Can you work these out from the model? Positions are in its coordinate system, mm. Face numbers are marked on the shaded views. A direction names the side the tool comes from. Coordinates: 2 decimals unless noted, no trailing zeros. Order: outer loops, then holes, each group sorted by start corner. A loop starts at its lowest first (then second) coordinate and runs counter-clockwise, first axis right, second up. Notation, with made-up numbers: M 67,-24 L 86,-24 A32 cw 86,6 Z; hole C 0,-2 d4. An arc over 180 degrees is marked long. Answer as a JSON object with one key per item and string values.
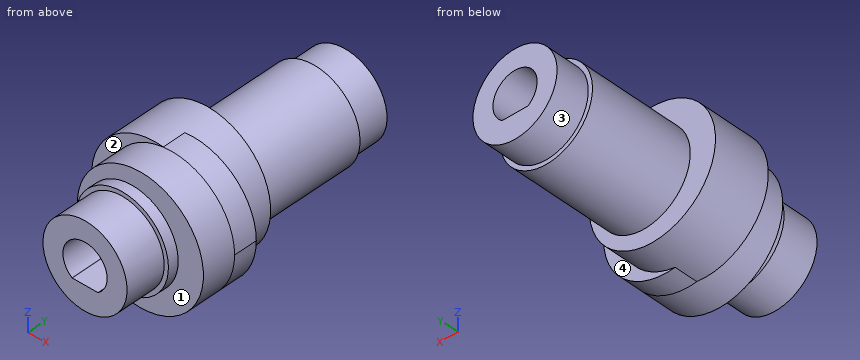
from build123d import *

# Parameters (mm, degrees)
SKETCH1_R            = 7.5
BOSS_EXTRUDE1_DEPTH  = 6.779166667
BOSS_EXTRUDE2_DEPTH  = 2.779166667
BOSS_EXTRUDE3_START  = -4
SKETCH1_4_R          = 7.5
BOSS_EXTRUDE3_DEPTH  = 4
BOSS_EXTRUDE4_START  = 6.016666667
SKETCH2_R            = 5
BOSS_EXTRUDE4_DEPTH  = 6.016666667
BOSS_EXTRUDE5_START  = 1.254166667
SKETCH2_3_R          = 5.5
SKETCH2_3_R_2        = 5
BOSS_EXTRUDE5_DEPTH  = 1.254166667
SKETCH3_R            = 5
BOSS_EXTRUDE9_DEPTH  = 16.541666667
SKETCH3_3_R          = 5.5
SKETCH3_3_R_2        = 5
BOSS_EXTRUDE10_DEPTH = 12.541666667


with BuildPart() as part:
    # Sketch1 → Boss-Extrude1 (new body)
    with BuildSketch(Plane(origin=(0, 0, 0), x_dir=(1, 0, 0), z_dir=(0, 1, 0))):
        with Locations(Location((-1, 0, 0), (0, 0, 270))):
            Circle(SKETCH1_R)
        with BuildLine():
            Line((-1.54175225, 2.127), (1.54175225, 2.127))
            ThreePointArc((1.54175225, 2.127), (0, -2.627), (-1.54175225, 2.127))
        make_face(mode=Mode.SUBTRACT)
    extrude(amount=BOSS_EXTRUDE1_DEPTH)

    # Sketch1<3> → Boss-Extrude2 (add)
    with BuildSketch(Plane(origin=(0, 0, 0), x_dir=(1, 0, 0), z_dir=(0, 1, 0))):
        with BuildLine():
            ThreePointArc((0, -7.433034374), (5.937104415, -5.645794895), (8.5, 0))
            ThreePointArc((8.5, 0), (5.937104415, 5.645794895), (0, 7.433034374))
            ThreePointArc((0, 7.433034374), (4.645794895, 4.937104415), (6.5, 0))
            ThreePointArc((6.5, 0), (4.645794895, -4.937104415), (0, -7.433034374))
        make_face()
    extrude(amount=BOSS_EXTRUDE2_DEPTH)

    # Sketch1<4> → Boss-Extrude3 (add)
    with BuildSketch(Plane(origin=(0, 0, 0), x_dir=(1, 0, 0), z_dir=(0, 1, 0)).offset(BOSS_EXTRUDE3_START)):
        with Locations(Location((1, 0, 0), (0, 0, 97.662255661))):
            Circle(SKETCH1_4_R)
        with BuildLine():
            Line((-1.54175225, 2.127), (1.54175225, 2.127))
            ThreePointArc((1.54175225, 2.127), (0, -2.627), (-1.54175225, 2.127))
        make_face(mode=Mode.SUBTRACT)
    extrude(amount=BOSS_EXTRUDE3_DEPTH)

    # Sketch2 → Boss-Extrude4 (add)
    with BuildSketch(Plane.XZ.offset(4).offset(BOSS_EXTRUDE4_START)):
        with Locations(Location((0, 0, 0), (0, 0, 90))):
            Circle(SKETCH2_R)
        with BuildLine():
            ThreePointArc((-1.54175225, -2.127), (0, 2.627), (1.54175225, -2.127))
            Line((1.54175225, -2.127), (-1.54175225, -2.127))
        make_face(mode=Mode.SUBTRACT)
    extrude(amount=-BOSS_EXTRUDE4_DEPTH)

    # Sketch2<3> → Boss-Extrude5 (add)
    with BuildSketch(Plane.XZ.offset(4).offset(BOSS_EXTRUDE5_START)):
        with Locations(Location((0, 0, 0), (0, 0, 90))):
            Circle(SKETCH2_3_R)
        with Locations(Location((0, 0, 0), (0, 0, 270))):
            Circle(SKETCH2_3_R_2, mode=Mode.SUBTRACT)
    extrude(amount=-BOSS_EXTRUDE5_DEPTH)

    # Sketch3 → Boss-Extrude9 (add)
    with BuildSketch(Plane(origin=(0, 6.779166667, 0), x_dir=(1, 0, 0), z_dir=(0, 1, 0))):
        with Locations(Location((0, 0, 0), (0, 0, 90))):
            Circle(SKETCH3_R)
        with BuildLine():
            Line((-1.54175225, 2.127), (1.54175225, 2.127))
            ThreePointArc((1.54175225, 2.127), (0, -2.627), (-1.54175225, 2.127))
        make_face(mode=Mode.SUBTRACT)
    extrude(amount=BOSS_EXTRUDE9_DEPTH)

    # Sketch3<3> → Boss-Extrude10 (add)
    with BuildSketch(Plane(origin=(0, 6.779166667, 0), x_dir=(1, 0, 0), z_dir=(0, 1, 0))):
        with Locations(Location((0, 0, 0), (0, 0, 270))):
            Circle(SKETCH3_3_R)
        with Locations(Location((0, 0, 0), (0, 0, 90))):
            Circle(SKETCH3_3_R_2, mode=Mode.SUBTRACT)
    extrude(amount=BOSS_EXTRUDE10_DEPTH)


solid = part.part
Item 1: Which directions (+Z, -Z, +X, -X, +Y, -Y) give clear straight access to the entire face, cutting with the end or side of a thin tool? Please do the marked faces 1, 2, 3 and 4.
Answers follow:
{"face 1": "-Y", "face 2": "-X, -Y", "face 3": "+Y", "face 4": "+X, +Y"}
Item 2: Please list where these lines run through material, in increasing order: line 1 (Z direction, x = 0, y = -5.75); line 2 (X direction, y = 2.5, z = 0); line 3 (Y direction, x = -7, z = 4.25).
Answers follow:
{"line 1": "z = -5 to -2.13, 2.63 to 5", "line 2": "x = -8.5 to -2.63, 2.63 to 8.5", "line 3": "y = 0 to 6.78"}
Item 3: I'm going to push flat-ended pins straight in: pin 1 (5.5 mm diameter, centred on x = 2.5, z = -0.5, fed in from -Y); pin 2 (1.5 mm diameter, centred on x = -2.5, y = 4.5, fed in from +Z); pin 3 (1.5 mm diameter, centred on x = 6.5, y = 3, fed in from -Z); pin 4 (1 mm diameter, centred on x = -5.5, z = -1.5, fed in from +Y). Where does each tip first touch, or does it pass through?
Answers follow:
{"pin 1": "stops at y = -10.02", "pin 2": "stops at z = 7.46", "pin 3": "stops at z = -5.78", "pin 4": "stops at y = 19.32"}
Item 4: I want a section at D-D, the plane y = 1.5. Write out the boundary of the cut face in (x, z), plus the area to 3 significant figures.
Answers follow:
{"outline": "M 0,-7.43 A7.5 ccw long 0,7.43 A7.5 ccw long Z; hole M -1.54,-2.13 L 1.54,-2.13 A2.63 ccw long Z", "area": "186 mm^2"}
Item 5: I want a section at B-B, the plane x = -2. Write out the boundary of the cut face in (y, z), plus the area to 3 significant figures.
Answers follow:
{"outline": "M -10.02,-4.58 L -5.25,-4.58 L -5.25,-5.12 L -4,-5.12 L -4,-6.87 L 0,-6.87 L 0,-7.43 L 6.78,-7.43 L 6.78,-5.12 L 19.32,-5.12 L 19.32,-4.58 L 23.32,-4.58 L 23.32,-1.7 L -10.02,-1.7 Z; M -10.02,1.7 L 23.32,1.7 L 23.32,4.58 L 19.32,4.58 L 19.32,5.12 L 6.78,5.12 L 6.78,7.43 L 0,7.43 L 0,6.87 L -4,6.87 L -4,5.12 L -5.25,5.12 L -5.25,4.58 L -10.02,4.58 Z", "area": "264 mm^2"}
Item 6: I want a section at A-A, the plane z = 1.75. Write out the boundary of the cut face in (x, y), plus the area to 3 significant figures.
Answers follow:
{"outline": "M -8.29,0 L -6.29,0 L -6.29,-4 L -5.21,-4 L -5.21,-5.25 L -4.68,-5.25 L -4.68,-10.02 L -1.96,-10.02 L -1.96,23.32 L -4.68,23.32 L -4.68,19.32 L -5.21,19.32 L -5.21,6.78 L -8.29,6.78 Z; M 1.96,-10.02 L 4.68,-10.02 L 4.68,-5.25 L 5.21,-5.25 L 5.21,-4 L 8.29,-4 L 8.29,2.78 L 6.29,2.78 L 6.29,6.78 L 5.21,6.78 L 5.21,19.32 L 4.68,19.32 L 4.68,23.32 L 1.96,23.32 Z", "area": "258 mm^2"}
Item 7: I want a section at C-C, the plane z = 4.5. Write out the boundary of the cut face in (x, y), plus the area to 3 significant figures.
Answers follow:
{"outline": "M -7,0 L -5,0 L -5,-4 L -3.16,-4 L -3.16,-5.25 L -2.18,-5.25 L -2.18,-10.02 L 2.18,-10.02 L 2.18,-5.25 L 3.16,-5.25 L 3.16,-4 L 7,-4 L 7,2.78 L 5,2.78 L 5,6.78 L 3.16,6.78 L 3.16,19.32 L 2.18,19.32 L 2.18,23.32 L -2.18,23.32 L -2.18,19.32 L -3.16,19.32 L -3.16,6.78 L -7,6.78 Z", "area": "260 mm^2"}
